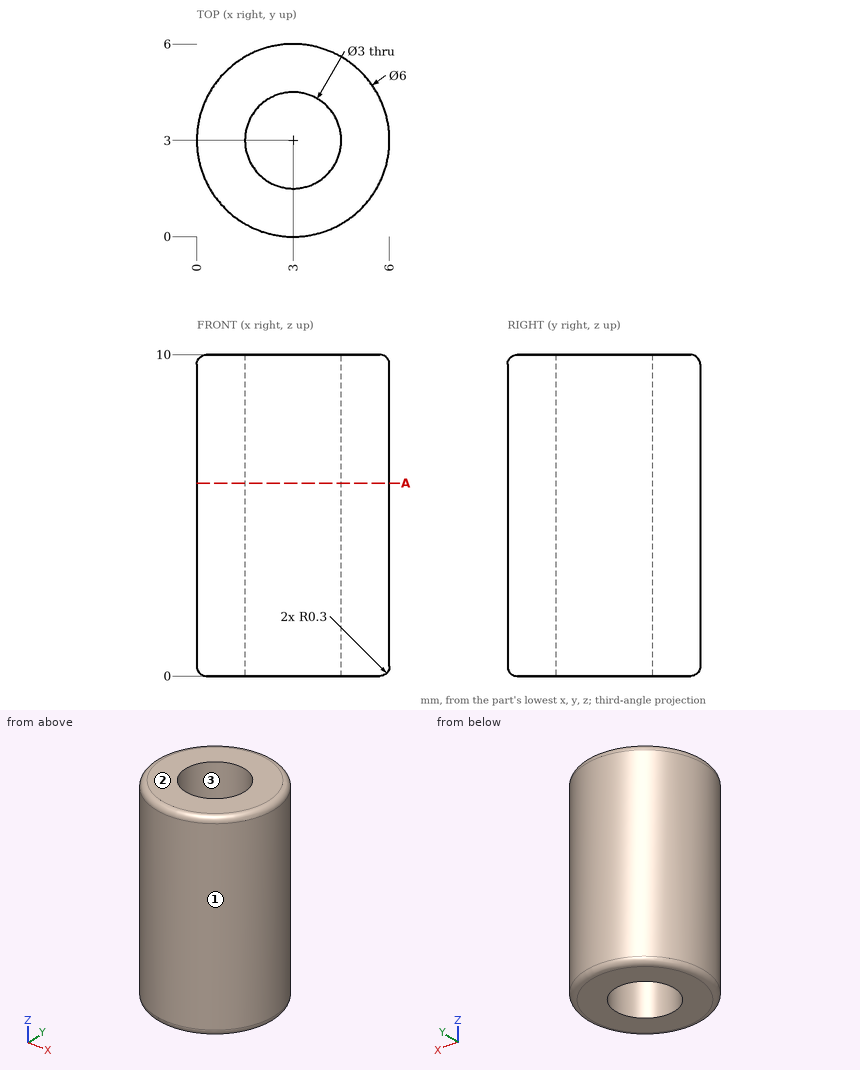
Part print with two shaded views. Sizes in mm from the minimum x, y, z corner. Round coordinates to 2 decimals unless told otherwise and drop trailing zeros. Order: outer loops, then holes, each group sorted by start corner. A loop starts at its lowest first (then second) coordinate and runs counter-clockwise, first axis right, second up. Notation, with made-up numbers: (8.25, 23.25) - (36.25, 23.25) arc R33 ccw to (36.25, 56.25) - close; hole circle Ø7 at (78, 52). An arc over 180 degrees is marked (long way). Return JSON: item names as keys, results as strings.
(1) Pull direction Y, two halves, no side cores. Call the marked faces 1, 2 and 3: +Y half, -Y half, draft (parallel to the pull), parting line (faces both ways), or undercut.
Answer key:
{"face 1": "parting line", "face 2": "draft", "face 3": "undercut"}
(2) Wall check: probe 1 along Y at (x, z) = (3, 6.75); probe 2 along X at (y, z) = (4, 6); probe 3 along Y at (x, z) = (1.25, 7.5). Give the ranges that are in metal, low to high. Write a range as from..to.
Answer key:
{"probe 1": "y = 0..1.5, 4.5..6", "probe 2": "x = 0.17..1.88, 4.12..5.83", "probe 3": "y = 0.56..5.44"}
(3) Pin check, flat tip, straight feed: pin 1 Ø2.5 at (x, y) = (3, 3) entering from +Z. Stop position of the tip, or through.
Answer key:
{"pin 1": "passes through"}
(4) Cut at A-A (z = 6). Give the cut face in (x, y).
Answer key:
{"outline": "circle Ø6 at (3, 3); hole circle Ø3 at (3, 3)"}
